Design review of the part built by this model. Coordinates are the model's own, in mm. Give positions to 0.01 mm unless a question says otherwise; leave off trailing zeros. Loops run counter-clockwise (first coordinate to the right, second up) from the corner with the lowest first, then second, coordinate; pieces in that order, holes last. Notation, with made-up numbers: M -8,66 L 23,66 A16 cw 23,97 Z; hole C 10.5,-22.75 d6. An arc over 180 degrees is marked long. Use a Markdown table: item, result. Add a question column.
(1) Insertion check: pin 1 Ø0.9 at (x, z) = (-42, 2) entering from -Y; pin 2 Ø1.5 at (y, z) = (-40, 2) entering from -X; pin 3 Ø0.9 at (y, z) = (40, 1.5) entering from +X. Each pin has a flat end and moves straight along its axis. Give the tip position at first contact, or say it passes through.
(2) For probe 1 along X at (y, z) = (-19.05, 2.05); probe 2 along Y at (x, z) = (43, 2.65); probe 3 along X at (y, z) = (31.5, 1.5), list the stretches that pass through material, from the lowest coordinate up.
(3) Add section B-B, the plane x = -6.5. Give the boundary of the cut face in (y, z), then the cut area to 3 significant figures.
(4) Add section A-A, the plane y = -6. Give the boundary of the cut face in (x, z).
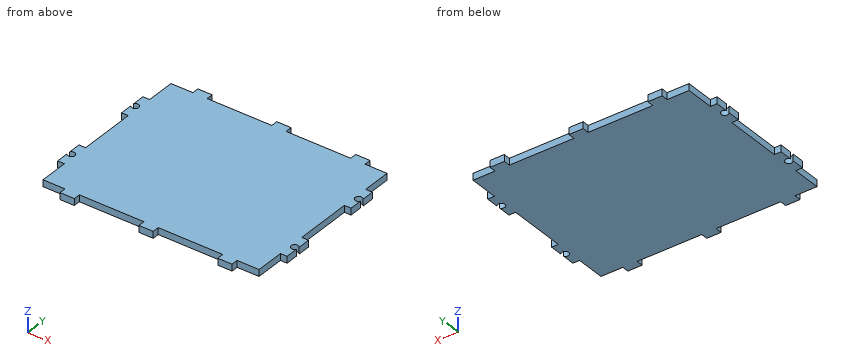
```python
from build123d import *

# Parameters (mm, degrees)
F1_DEPTH = 2.9718


with BuildPart() as f1:
    # F0 (on Top) → F1 (new body)
    with BuildSketch(Plane.XY):
        with BuildLine():
            Line((47.8282, 25.4), (47.8282, 38.1))
            Line((47.8282, 38.1), (38.1, 38.1))
            Line((38.1, 38.1), (38.1, 41.0718))
            Line((38.1, 41.0718), (31.75, 41.0718))
            Line((31.75, 41.0718), (31.75, 38.1))
            Line((31.75, 38.1), (3.175, 38.1))
            Line((3.175, 38.1), (3.175, 41.0718))
            Line((3.175, 41.0718), (-3.175, 41.0718))
            Line((-3.175, 41.0718), (-3.175, 38.1))
            Line((-3.175, 38.1), (-31.75, 38.1))
            Line((-31.75, 38.1), (-31.75, 41.0718))
            Line((-31.75, 41.0718), (-38.1, 41.0718))
            Line((-38.1, 41.0718), (-38.1, 38.1))
            Line((-38.1, 38.1), (-47.8282, 38.1))
            Line((-47.8282, 38.1), (-47.8282, 25.4))
            Line((-47.8282, 25.4), (-50.8, 25.4))
            Line((-50.8, 25.4), (-50.8, 19.891369))
            ThreePointArc((-50.8, 19.891369), (-47.8663, 19.05), (-50.8, 18.208631))
            Line((-50.8, 18.208631), (-50.8, 12.7))
            Line((-50.8, 12.7), (-47.8282, 12.7))
            Line((-47.8282, 12.7), (-47.8282, 0))
            Line((-47.8282, 0), (-47.8282, -12.7))
            Line((-47.8282, -12.7), (-50.8, -12.7))
            Line((-50.8, -12.7), (-50.8, -18.208631))
            ThreePointArc((-50.8, -18.208631), (-47.8663, -19.05), (-50.8, -19.891369))
            Line((-50.8, -19.891369), (-50.8, -25.4))
            Line((-50.8, -25.4), (-47.8282, -25.4))
            Line((-47.8282, -25.4), (-47.8282, -38.1))
            Line((-47.8282, -38.1), (-38.1, -38.1))
            Line((-38.1, -38.1), (-38.1, -41.0718))
            Line((-38.1, -41.0718), (-31.75, -41.0718))
            Line((-31.75, -41.0718), (-31.75, -38.1))
            Line((-31.75, -38.1), (-3.175, -38.1))
            Line((-3.175, -38.1), (-3.175, -41.0718))
            Line((-3.175, -41.0718), (3.175, -41.0718))
            Line((3.175, -41.0718), (3.175, -38.1))
            Line((3.175, -38.1), (31.75, -38.1))
            Line((31.75, -38.1), (31.75, -41.0718))
            Line((31.75, -41.0718), (38.1, -41.0718))
            Line((38.1, -41.0718), (38.1, -38.1))
            Line((38.1, -38.1), (47.8282, -38.1))
            Line((47.8282, -38.1), (47.8282, -25.4))
            Line((47.8282, -25.4), (50.8, -25.4))
            Line((50.8, -25.4), (50.8, -19.891369))
            ThreePointArc((50.8, -19.891369), (47.8663, -19.05), (50.8, -18.208631))
            Line((50.8, -18.208631), (50.8, -12.7))
            Line((50.8, -12.7), (47.8282, -12.7))
            Line((47.8282, -12.7), (47.8282, 0))
            Line((47.8282, 0), (47.8282, 12.7))
            Line((47.8282, 12.7), (50.8, 12.7))
            Line((50.8, 12.7), (50.8, 18.208631))
            ThreePointArc((50.8, 18.208631), (47.8663, 19.05), (50.8, 19.891369))
            Line((50.8, 19.891369), (50.8, 25.4))
            Line((50.8, 25.4), (47.8282, 25.4))
        make_face()
    extrude(amount=F1_DEPTH)


solid = f1.part
```
Established:
| question | item | result |
|---|---|---|
| 1 | pin 1 | y = -38.1 |
| 1 | pin 2 | x = -38.1 |
| 1 | pin 3 | x = 38.1 |
| 2 | probe 1 | -47.87 to 47.87 |
| 2 | probe 2 | -38.1 to 38.1 |
| 2 | probe 3 | -47.83 to 47.83 |
| 3 | outline | M -38.1,0 L 38.1,0 L 38.1,2.97 L -38.1,2.97 Z |
| 3 | area | 226 mm^2 |
| 4 | outline | M -47.83,0 L 47.83,0 L 47.83,2.97 L -47.83,2.97 Z |
